from build123d import *

# Parameters (mm, degrees)
SKETCH1_W           = 127
SKETCH1_H           = 63.5
BOSS_EXTRUDE1_DEPTH = 88.9
SKETCH3_R           = 63.5
BOSS_EXTRUDE2_DEPTH = 139.7
CUT_EXTRUDE1_REACH  = 213.465
CUT_EXTRUDE2_REACH  = 213.465
SKETCH5_R           = 38.1


with BuildPart() as part:
    # Sketch1 → Boss-Extrude1 (new body)
    with BuildSketch(Plane(origin=(0, 0, 0), x_dir=(1, 0, 0), z_dir=(0, 1, 0))):
        with Locations((63.5, 31.75)):
            Rectangle(SKETCH1_W, SKETCH1_H)
    extrude(amount=BOSS_EXTRUDE1_DEPTH)

    # Sketch3 → Boss-Extrude2 (add)
    with BuildSketch(Plane.XZ):
        with Locations(Location((0, -31.75, 0), (0, 0, 270))):
            Circle(SKETCH3_R)
    extrude(amount=-BOSS_EXTRUDE2_DEPTH)

    # Sketch4 → Cut-Extrude1 (cut, up to next)
    with BuildSketch(Plane.XY, mode=Mode.PRIVATE) as cut_extrude1_sk1:
        Polygon((82.55, 88.9), (127, 44.45), (127, 88.9), align=None)
    cut_extrude1_tool1 = extrude(cut_extrude1_sk1.sketch, amount=-CUT_EXTRUDE1_REACH, mode=Mode.PRIVATE) & part.part
    add(cut_extrude1_tool1.solids().sort_by_distance((112.183333, 74.083333, 0))[0], mode=Mode.SUBTRACT)

    # Sketch5 → Cut-Extrude2 (cut, up to next)
    with BuildSketch(Plane(origin=(0, 139.7, 0), x_dir=(1, 0, 0), z_dir=(0, 1, 0)), mode=Mode.PRIVATE) as cut_extrude2_sk1:
        with Locations(Location((0, 31.75, 0), (0, 0, 270))):
            Circle(SKETCH5_R)
    cut_extrude2_tool1 = extrude(cut_extrude2_sk1.sketch, amount=-CUT_EXTRUDE2_REACH, mode=Mode.PRIVATE) & part.part
    add(cut_extrude2_tool1.solids().sort_by_distance((0, 139.7, -31.75))[0], mode=Mode.SUBTRACT)


solid = part.part
Part model, mm, in its own coordinate system. A direction names the side the tool comes from. Coordinates: 2 decimals unless noted, no trailing zeros. Order: outer loops, then holes, each group sorted by start corner. A loop starts at its lowest first (then second) coordinate and runs counter-clockwise, first axis right, second up. Notation, with made-up numbers: M 4,67.25 L 32,67.25 A12 ccw 32,71.25 Z; hole C -0.75,-20.75 d2. An arc over 180 degrees is marked long. One line per question, with ' | ' between items.
Q1. Slice it at D-D (z = -31.75). Give the cut face in (x, y), and give its area (3 significant figures).
A:
outline: M -63.5,0 L -38.1,0 L -38.1,139.7 L -63.5,139.7 Z; M 38.1,0 L 127,0 L 127,44.45 L 82.55,88.9 L 63.5,88.9 L 63.5,139.7 L 38.1,139.7 Z | area: 11,800 mm^2
Q2. Two-plate mould, pull along Z, no slides. Class faces 3 (the face through (-61.99, 68.87, -17.98)), 4 (the face through (104.46, 66.99, -31.31)), 5 (the face through (90, 34, 0)), 6 (the face through (11.44, 70.83, 4.59)): +Z half, -Z half, draft (parallel to the pull), parting line (faces both ways), or undercut.
A:
face 3: parting line | face 4: draft | face 5: +Z half | face 6: undercut
Q3. Pin check, flat tips, straight feed: P1, Ø1.5, axis at y = 79, z = -1.5, coming from the +X side; P2, Ø12, axis at x = 36, y = 87, coming from the -Z side; P3, Ø4, axis at y = 82, z = 0.5, coming from the -X side; P4, Ø22, axis at x = 63.5, z = -16.5, coming from the +Y side. Stop position of each tip, or through.
A:
P1: stops at x = 93.2 | P2: stops at z = -87.72 | P3: stops at x = -55.83 | P4: stops at y = 139.7
Q4. Slice it at A-A (x = 0). Give the cut face in (y, z), and give its area (3 significant figures).
A:
outline: M 0,-95.25 L 139.7,-95.25 L 139.7,-69.85 L 0,-69.85 Z; M 0,6.35 L 139.7,6.35 L 139.7,31.75 L 0,31.75 Z | area: 7,100 mm^2
Q5. Slice it at B-B (y = 19.5). Give the cut face in (x, z).
A:
outline: M 54.99,-63.5 L 127,-63.5 L 127,0 L 54.99,0 A63.5 ccw long Z; hole C 0,-31.75 d76.2
Q6. Drill centre lines: line 1 (X direction, y = 106.5, z = -30.5); line 2 (X direction, y = 31, z = -31.75); line 3 (Y direction, x = 81, z = -34). Where is each one in solid material? Low to high.
A:
line 1: x = -63.49 to -38.08, 38.08 to 63.49 | line 2: x = -63.5 to -38.1, 38.1 to 127 | line 3: y = 0 to 88.9
Q7. 3-axis set-ups, long thin cutter, end or side, ignore diameter. For faces 1 (the face through (-27, 139.7, -59)), 2 (the face through (90, 34, -63.5)): which of +Z, -Z, +X, -X, +Y, -Y reach the whole face in a straight line?
A:
face 1: +Z, -Z, +X, -X, +Y | face 2: -Z, +X, +Y, -Y
Q8. Slice it at C-C (z = -15). Give the cut face in (x, y), and give its area (3 significant figures).
A:
outline: M -61.25,0 L -34.22,0 L -34.22,139.7 L -61.25,139.7 Z; M 34.22,0 L 127,0 L 127,44.45 L 82.55,88.9 L 61.25,88.9 L 61.25,139.7 L 34.22,139.7 Z | area: 12,400 mm^2
